Here's how the part is built. I have some questions about the finished solid (model axes, mm). Face numbers are marked on the shaded views. A direction names the side the tool comes from. Round coordinates to 2 decimals unless told otherwise and drop trailing zeros. Write each loop counter-clockwise with the first axis right and the second up, starting at its lowest first coordinate (ties: lowest second). Pieces come first, ordered by that corner, then holes. Notation, with made-up numbers: (-18.5, 43) - (21.5, 43) arc R25 ccw to (21.5, 58) - close; hole circle Ø3 at (-36, 63). An arc over 180 degrees is marked (long way). One line per question, with ' | ' between items. Start each with the question number.
(1) If I drill on L1, parallel to Z at x = -43.5, y = 1.75; L2, parallel to Z at x = 9, y = 5.25; L3, parallel to Y at x = -52.25, z = -21, over which ranges is the centre line in solid material (lowest first)?
(2) Thinking about a two-plate mould opening in X: for the marked faces 3, 4 and 5, which applies, pulls with the +X half, pulls with the -X half, needs draft (parallel to the pull), parting line crosses it, or undercut?
(3) For the marked faces 1 and 2, which set-ups out of +Z, -Z, +X, -X, +Y, -Y let a thin tool reach every point of the face, with its end or its side?
(4) Imagine slicing it at B-B (x = 7.5). Write out the boundary of the cut face in (y, z).
(5) Imagine slicing it at A-A (x = 40). Write out the boundary of the cut face in (y, z), plus the area to 3 significant figures.
(6) Will these pins go through, and if not, where does the flat tip stop? pin 1 (2 mm diameter, centred on x = -22.5, y = 5, fed in from +Z); pin 2 (1.3 mm diameter, centred on x = -7.5, y = 4.5, fed in from -Z); pin 3 (2 mm diameter, centred on y = 5, z = -21, fed in from -X).
(7) Imagine slicing it at C-C (y = 2). Give the number of separate pieces and of enclosed holes in the cut face, plus the area to 3 significant figures.
from build123d import *

# Parameters (mm, degrees)
SKETCH_1_W               = 114
SKETCH_1_H               = 72.5
EXTRUDE_1_DEPTH          = 10
SKETCH_2_R               = 1.3
CUT_EXTRUDE_1_DEPTH      = 8
PATTERN_LINEAR_1_COUNT   = 4
PATTERN_LINEAR_1_PITCH   = 15
MIRROR_1_COPY_1_SKETCH_R = 1.3
MIRROR_1_COPY_1_DEPTH    = 8
MIRROR_1_COPY_2_SKETCH_R = 1.3
MIRROR_1_COPY_2_DEPTH    = 8
MIRROR_1_COPY_3_SKETCH_R = 1.3
MIRROR_1_COPY_3_DEPTH    = 8
SKETCH_3_R               = 1.3
CUT_EXTRUDE_2_DEPTH      = 7.5
PATTERN_LINEAR_2_COUNT   = 4
PATTERN_LINEAR_2_PITCH   = 14
MIRROR_2_COPY_1_SKETCH_R = 1.3
MIRROR_2_COPY_1_DEPTH    = 7.5
MIRROR_2_COPY_2_SKETCH_R = 1.3
MIRROR_2_COPY_2_DEPTH    = 7.5
MIRROR_2_COPY_3_SKETCH_R = 1.3
MIRROR_2_COPY_3_DEPTH    = 7.5
CUT_EXTRUDE_3_REACH      = 70.287
SKETCH_4_W               = 13
SKETCH_4_H               = 20
FILLET_1_R               = 2
CHAMFER_1_SIZE           = 0.2


with BuildPart() as part:
    # 草圖1 → 填料-伸長1 (new body)
    with BuildSketch(Plane(origin=(0, 0, 0), x_dir=(1, 0, 0), z_dir=(0, 1, 0))):
        Rectangle(SKETCH_1_W, SKETCH_1_H)
    extrude(amount=EXTRUDE_1_DEPTH)

    # 草圖2 → 除料-伸長1 (cut)
    with BuildSketch(Plane.XY.offset(36.25)):
        with Locations((-22.5, 5)):
            Circle(SKETCH_2_R)
    cut_extrude_1 = extrude(amount=-CUT_EXTRUDE_1_DEPTH, mode=Mode.SUBTRACT)

    # 直線複製排列1: 除料-伸長1 ×4
    with Locations(*[(i * PATTERN_LINEAR_1_PITCH, 0, 0) for i in range(1, PATTERN_LINEAR_1_COUNT)]):
        add(cut_extrude_1, mode=Mode.SUBTRACT)

    # 鏡射1: 除料-伸長1 across plane
    add(cut_extrude_1.mirror(Plane.XY), mode=Mode.SUBTRACT)

    # 鏡射1 copy 1 sketch → 鏡射1 copy 1 (cut)
    with BuildSketch(Plane(origin=(15, 0, -36.25), x_dir=(1, 0, 0), z_dir=(0, 0, -1))):
        with Locations((-22.5, -5)):
            Circle(MIRROR_1_COPY_1_SKETCH_R)
    extrude(amount=-MIRROR_1_COPY_1_DEPTH, mode=Mode.SUBTRACT)

    # 鏡射1 copy 2 sketch → 鏡射1 copy 2 (cut)
    with BuildSketch(Plane(origin=(30, 0, -36.25), x_dir=(1, 0, 0), z_dir=(0, 0, -1))):
        with Locations((-22.5, -5)):
            Circle(MIRROR_1_COPY_2_SKETCH_R)
    extrude(amount=-MIRROR_1_COPY_2_DEPTH, mode=Mode.SUBTRACT)

    # 鏡射1 copy 3 sketch → 鏡射1 copy 3 (cut)
    with BuildSketch(Plane(origin=(45, 0, -36.25), x_dir=(1, 0, 0), z_dir=(0, 0, -1))):
        with Locations((-22.5, -5)):
            Circle(MIRROR_1_COPY_3_SKETCH_R)
    extrude(amount=-MIRROR_1_COPY_3_DEPTH, mode=Mode.SUBTRACT)

    # 草圖3 → 除料-伸長2 (cut)
    with BuildSketch(Plane.ZY.offset(57)):
        with Locations((-21, 5)):
            Circle(SKETCH_3_R)
    cut_extrude_2 = extrude(amount=-CUT_EXTRUDE_2_DEPTH, mode=Mode.SUBTRACT)

    # 直線複製排列2: 除料-伸長2 ×4
    with Locations(*[(0, 0, i * PATTERN_LINEAR_2_PITCH) for i in range(1, PATTERN_LINEAR_2_COUNT)]):
        add(cut_extrude_2, mode=Mode.SUBTRACT)

    # 鏡射2: 除料-伸長2 across plane
    add(cut_extrude_2.mirror(Plane(origin=(0, 0, 0), x_dir=(0, 0, 1), z_dir=(1, 0, 0))), mode=Mode.SUBTRACT)

    # 鏡射2 copy 1 sketch → 鏡射2 copy 1 (cut)
    with BuildSketch(Plane(origin=(57, 0, 14), x_dir=(0, 0, 1), z_dir=(1, 0, 0))):
        with Locations((-21, -5)):
            Circle(MIRROR_2_COPY_1_SKETCH_R)
    extrude(amount=-MIRROR_2_COPY_1_DEPTH, mode=Mode.SUBTRACT)

    # 鏡射2 copy 2 sketch → 鏡射2 copy 2 (cut)
    with BuildSketch(Plane(origin=(57, 0, 28), x_dir=(0, 0, 1), z_dir=(1, 0, 0))):
        with Locations((-21, -5)):
            Circle(MIRROR_2_COPY_2_SKETCH_R)
    extrude(amount=-MIRROR_2_COPY_2_DEPTH, mode=Mode.SUBTRACT)

    # 鏡射2 copy 3 sketch → 鏡射2 copy 3 (cut)
    with BuildSketch(Plane(origin=(57, 0, 42), x_dir=(0, 0, 1), z_dir=(1, 0, 0))):
        with Locations((-21, -5)):
            Circle(MIRROR_2_COPY_3_SKETCH_R)
    extrude(amount=-MIRROR_2_COPY_3_DEPTH, mode=Mode.SUBTRACT)

    # 草圖4 → 除料-伸長3 (cut, up to next)
    with BuildSketch(Plane(origin=(0, 10, 0), x_dir=(1, 0, 0), z_dir=(0, 1, 0)), mode=Mode.PRIVATE) as cut_extrude_3_sk1:
        Polygon((-45.5, 18.967619242), (-45.5, -18.967619242), (-13.887301263, 0), align=None)
    cut_extrude_3_tool1 = extrude(cut_extrude_3_sk1.sketch, amount=-CUT_EXTRUDE_3_REACH, mode=Mode.PRIVATE) & part.part
    # 草圖4 → 除料-伸長3 (cut, up to next)
    with BuildSketch(Plane(origin=(0, 10, 0), x_dir=(1, 0, 0), z_dir=(0, 1, 0)), mode=Mode.PRIVATE) as cut_extrude_3_sk2:
        Polygon((-40.279365403, 20.5), (-10, 2.332380758), (20.279365403, 20.5), align=None)
    cut_extrude_3_tool2 = extrude(cut_extrude_3_sk2.sketch, amount=-CUT_EXTRUDE_3_REACH, mode=Mode.PRIVATE) & part.part
    # 草圖4 → 除料-伸長3 (cut, up to next)
    with BuildSketch(Plane(origin=(0, 10, 0), x_dir=(1, 0, 0), z_dir=(0, 1, 0)), mode=Mode.PRIVATE) as cut_extrude_3_sk3:
        Polygon((-6.112698737, 0), (25.5, 18.967619242), (25.5, -18.967619242), align=None)
    cut_extrude_3_tool3 = extrude(cut_extrude_3_sk3.sketch, amount=-CUT_EXTRUDE_3_REACH, mode=Mode.PRIVATE) & part.part
    # 草圖4 → 除料-伸長3 (cut, up to next)
    with BuildSketch(Plane(origin=(0, 10, 0), x_dir=(1, 0, 0), z_dir=(0, 1, 0)), mode=Mode.PRIVATE) as cut_extrude_3_sk4:
        Polygon((-10, -2.332380758), (20.279365403, -20.5), (-40.279365403, -20.5), align=None)
    cut_extrude_3_tool4 = extrude(cut_extrude_3_sk4.sketch, amount=-CUT_EXTRUDE_3_REACH, mode=Mode.PRIVATE) & part.part
    # 草圖4 → 除料-伸長3 (cut, up to next)
    with BuildSketch(Plane(origin=(0, 10, 0), x_dir=(1, 0, 0), z_dir=(0, 1, 0)), mode=Mode.PRIVATE) as cut_extrude_3_sk5:
        with Locations((40.5, 0)):
            Rectangle(SKETCH_4_W, SKETCH_4_H)
    cut_extrude_3_tool5 = extrude(cut_extrude_3_sk5.sketch, amount=-CUT_EXTRUDE_3_REACH, mode=Mode.PRIVATE) & part.part
    add(cut_extrude_3_tool1.solids().sort_by_distance((-34.962434, 10, 0))[0], mode=Mode.SUBTRACT)
    add(cut_extrude_3_tool2.solids().sort_by_distance((-10, 10, -14.444127))[0], mode=Mode.SUBTRACT)
    add(cut_extrude_3_tool3.solids().sort_by_distance((14.962434, 10, 0))[0], mode=Mode.SUBTRACT)
    add(cut_extrude_3_tool4.solids().sort_by_distance((-10, 10, 14.444127))[0], mode=Mode.SUBTRACT)
    add(cut_extrude_3_tool5.solids().sort_by_distance((40.5, 10, 0))[0], mode=Mode.SUBTRACT)

    # 圓角1
    fillet_1_edges = [part.edges().sort_by_distance(p)[0] for p in [
        (-45.5, 5, 18.967619242),
        (-45.5, 5, -18.967619242),
        (-13.887301263, 5, 0),
        (-6.112698737, 5, 0),
        (25.5, 5, -18.967619242),
        (25.5, 5, 18.967619242),
        (-10, 5, -2.332380758),
        (-40.279365403, 5, -20.5),
        (20.279365403, 5, -20.5),
        (-10, 5, 2.332380758),
        (20.279365403, 5, 20.5),
        (-40.279365403, 5, 20.5),
        (47, 5, -10),
        (47, 5, 10),
        (34, 5, 10),
        (34, 5, -10),
    ]]
    fillet(fillet_1_edges, radius=FILLET_1_R)

    # 導角1
    chamfer_1_edges = [part.edges().sort_by_distance(p)[0] for p in [
        (-23.8, 5, 36.25),
        (-8.8, 5, 36.25),
        (6.2, 5, 36.25),
        (21.2, 5, 36.25),
        (-23.8, 5, -36.25),
        (-8.8, 5, -36.25),
        (6.2, 5, -36.25),
        (21.2, 5, -36.25),
        (-57, 5, -22.3),
        (-57, 5, -8.3),
        (-57, 5, 5.7),
        (-57, 5, 19.7),
        (57, 5, -22.3),
        (57, 5, -8.3),
        (57, 5, 5.7),
        (57, 5, 19.7),
    ]]
    chamfer(chamfer_1_edges, length=CHAMFER_1_SIZE)


solid = part.part
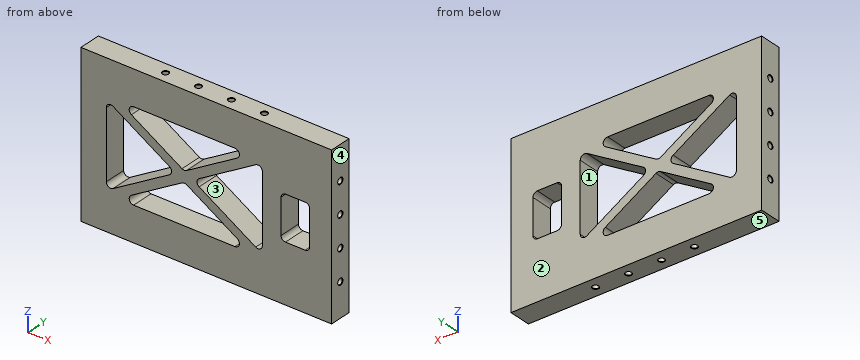
Check sheet entries:
1) L1: -36.25 to -17.44, 17.44 to 36.25 | L2: -36.25 to -20.5, -13.73 to -9.07, 9.07 to 13.73, 20.5 to 36.25 | L3: 0 to 3.7, 6.3 to 10
2) face 3: undercut | face 4: pulls with the +X half | face 5: needs draft
3) face 1: +Y, -Y | face 2: +Z, -Z, +X, -X, +Y
4) outline: (0, -36.25) - (3.5, -36.25) - (3.7, -36.05) - (3.7, -28.25) - (6.3, -28.25) - (6.3, -36.05) - (6.5, -36.25) - (10, -36.25) - (10, -20.5) - (0, -20.5) - close; (0, -12.83) - (10, -12.83) - (10, -8.17) - (0, -8.17) - close; (0, 8.17) - (10, 8.17) - (10, 12.83) - (0, 12.83) - close; (0, 20.5) - (10, 20.5) - (10, 36.25) - (6.5, 36.25) - (6.3, 36.05) - (6.3, 28.25) - (3.7, 28.25) - (3.7, 36.05) - (3.5, 36.25) - (0, 36.25) - close
5) outline: (0, -36.25) - (10, -36.25) - (10, -10) - (0, -10) - close; (0, 10) - (10, 10) - (10, 36.25) - (0, 36.25) - close | area: 525 mm^2
6) pin 1: z = 28.25 | pin 2: z = -28.25 | pin 3: x = -49.5
7) separate pieces: 1 | enclosed holes: 5 | area: 5,760 mm^2
